Part model, mm, in its own coordinate system. Give positions to 0.01 mm unless a question says otherwise; leave off trailing zeros. Order: outer loops, then holes, each group sorted by start corner. A loop starts at its lowest first (then second) coordinate and runs counter-clockwise, first axis right, second up.
1. Slice it at C-C on x = 782. List the corners of the cut face in (y, z) (3 decimals).
2. Slice it at B-B on x = 1372.5. List the corners of the cut face in (y, z) (3 decimals), and give its area (3 significant figures).
3. Slice it at D-D on y = -6.25. Give the number of separate pieces and of enclosed holes in the cut face, and give its area (3 significant figures).
4. Drop a flat-ended pin along its axis: pin 1 Ø8 at (y, z) = (-14.5, 220) entering from -X. Give the stop position or say it passes through.
5. Slice it at A-A on z = 98. List the corners of the cut face in (x, y).
6. Probe line 1 (Z direction, x = 897.5, y = -13.75) (3 decimals); line 2 (X direction, y = -10.5, z = 375); line 3 (X direction, y = -10.5, z = 684.5). List the from-to ranges inside material, lowest first.
from build123d import *

# Parameters (mm, degrees)
F0_W     = 1524
F0_H     = 749.3
F0_W_2   = 533.4
F0_H_2   = 673.1
F0_W_3   = 304.8
F1_DEPTH = 19.05
F2_W     = 19.05
F2_H     = 38.1
F3_DEPTH = 1447.8
F4_W     = 19.05
F4_H     = 38.1
F5_DEPTH = 304.8
F6_W     = 19.05
F6_H     = 38.1
F7_DEPTH = 304.8


with BuildPart() as f1:
    # F0 (on Front) → F1 (new body)
    with BuildSketch(Plane.XZ):
        with Locations((762, 374.65)):
            Rectangle(F0_W, F0_H)
        with Locations((304.8, 374.65)):
            Rectangle(F0_W_2, F0_H_2, mode=Mode.SUBTRACT)
        with Locations((762, 374.65)):
            Rectangle(F0_W_3, F0_H_2, mode=Mode.SUBTRACT)
        with Locations((1219.2, 374.65)):
            Rectangle(F0_W_2, F0_H_2, mode=Mode.SUBTRACT)
    extrude(amount=F1_DEPTH)

    # F2 (on face) → F3 (join, through all)
    with BuildSketch(Plane.YZ.offset(38.1)):
        with Locations((-9.525, 561.975)):
            Rectangle(F2_W, F2_H)
    extrude(amount=F3_DEPTH)

    # F4 (on face) → F5 (join, through all)
    with BuildSketch(Plane.YZ.offset(609.6)):
        with Locations((-9.525, 377.825)):
            Rectangle(F4_W, F4_H)
    extrude(amount=F5_DEPTH)

    # F6 (on face) → F7 (join, through all)
    with BuildSketch(Plane.YZ.offset(609.6)):
        with Locations((-9.525, 193.675)):
            Rectangle(F6_W, F6_H)
    extrude(amount=F7_DEPTH)


solid = f1.part
Data:
1. outline: (-19.05, 0) - (0, 0) - (0, 38.1) - (-19.05, 38.1) - close; (-19.05, 174.625) - (0, 174.625) - (0, 212.725) - (-19.05, 212.725) - close; (-19.05, 358.775) - (0, 358.775) - (0, 396.875) - (-19.05, 396.875) - close; (-19.05, 542.925) - (0, 542.925) - (0, 581.025) - (-19.05, 581.025) - close; (-19.05, 711.2) - (0, 711.2) - (0, 749.3) - (-19.05, 749.3) - close
2. outline: (-19.05, 0) - (0, 0) - (0, 38.1) - (-19.05, 38.1) - close; (-19.05, 542.925) - (0, 542.925) - (0, 581.025) - (-19.05, 581.025) - close; (-19.05, 711.2) - (0, 711.2) - (0, 749.3) - (-19.05, 749.3) - close
2. area: 2,180 mm2
3. separate pieces: 1
3. enclosed holes: 8
3. area: 294,000 mm2
4. pin 1: stops at x = 0
5. outline: (0, -19.05) - (38.1, -19.05) - (38.1, 0) - (0, 0) - close; (571.5, -19.05) - (609.6, -19.05) - (609.6, 0) - (571.5, 0) - close; (914.4, -19.05) - (952.5, -19.05) - (952.5, 0) - (914.4, 0) - close; (1485.9, -19.05) - (1524, -19.05) - (1524, 0) - (1485.9, 0) - close
6. line 1: z = 0 to 38.1, 174.625 to 212.725, 358.775 to 396.875, 542.925 to 581.025, 711.2 to 749.3
6. line 2: x = 0 to 38.1, 571.5 to 952.5, 1485.9 to 1524
6. line 3: x = 0 to 38.1, 571.5 to 609.6, 914.4 to 952.5, 1485.9 to 1524
